```python
from build123d import *

# Parameters (mm, degrees)
BOSS_EXTRUDE1_DEPTH = 18
SKETCH2_R           = 1.75
CUT_EXTRUDE1_DEPTH  = 30.5
CUT_EXTRUDE2_DEPTH  = 1
CUT_EXTRUDE3_DEPTH  = 5


with BuildPart() as part:
    # Sketch1 → Boss-Extrude1 (new body)
    with BuildSketch(Plane(origin=(0, 0, 0), x_dir=(1, 0, 0), z_dir=(0, 1, 0))):
        with BuildLine():
            ThreePointArc((-16.998275301, 22.028571429), (-24.773162376, 20.985576383), (-31.998275301, 17.93034302))
            ThreePointArc((-31.998275301, 17.93034302), (-46.498275301, -7.471428571), (-31.998275301, -32.873200163))
            ThreePointArc((-31.998275301, -32.873200163), (-24.773162376, -35.928433526), (-16.998275301, -36.971428571))
            Line((-16.998275301, -36.971428571), (-16.998275301, -29.971428571))
            ThreePointArc((-16.998275301, -29.971428571), (-39.498275301, -7.471428571), (-16.998275301, 15.028571429))
            Line((-16.998275301, 15.028571429), (-16.998275301, 22.028571429))
        make_face()
        with BuildLine():
            Line((-16.998275301, 32.528571429), (-31.998275301, 32.528571429))
            Line((-31.998275301, 32.528571429), (-31.998275301, 17.93034302))
            ThreePointArc((-31.998275301, 17.93034302), (-24.773162376, 20.985576383), (-16.998275301, 22.028571429))
            Line((-16.998275301, 22.028571429), (-16.998275301, 32.528571429))
        make_face()
        with BuildLine():
            Line((-31.998275301, -32.873200163), (-31.998275301, -47.471428571))
            Line((-31.998275301, -47.471428571), (-16.998275301, -47.471428571))
            Line((-16.998275301, -47.471428571), (-16.998275301, -36.971428571))
            ThreePointArc((-16.998275301, -36.971428571), (-24.773162376, -35.928433526), (-31.998275301, -32.873200163))
        make_face()
    extrude(amount=BOSS_EXTRUDE1_DEPTH)

    # Sketch2 → Cut-Extrude1 (cut, through all)
    with BuildSketch(Plane(origin=(-16.998275301, 0, 0), x_dir=(0, 0, -1), z_dir=(1, 0, 0))):
        with Locations((-42.471428571, 5.25)):
            Circle(SKETCH2_R)
        with Locations((27.528571429, 5.25)):
            Circle(SKETCH2_R)
    extrude(amount=-CUT_EXTRUDE1_DEPTH, mode=Mode.SUBTRACT)

    # Sketch3 → Cut-Extrude2 (cut)
    with BuildSketch(Plane(origin=(-16.998275301, 0, 0), x_dir=(0, 0, -1), z_dir=(1, 0, 0))):
        Polygon((-40.05243206, 15.382896708), (-37.474440607, 15.382896708), (-37.474440607, 14.433110383), (-39.102645735, 14.433110383), (-39.102645735, 13.415482178), (-37.474440607, 13.415482178), (-37.474440607, 12.465695853), (-39.102645735, 12.465695853), (-39.102645735, 10.091230041), (-40.05243206, 10.091230041), align=None)
        Polygon((-35.957538563, 15.382896708), (-34.489397872, 15.382896708), (-34.489397872, 10.091230041), (-35.439184196, 10.091230041), (-35.439184196, 14.500952263), (-36.524654282, 14.500952263), align=None)
    extrude(amount=-CUT_EXTRUDE2_DEPTH, mode=Mode.SUBTRACT)

    # Sketch4 → Cut-Extrude3 (cut)
    with BuildSketch(Plane.ZY.offset(31.998275301)):
        Polygon((-26.308738524, 2.318218798), (-24.379657977, 4.840515682), (-25.599490881, 7.772296885), (-28.748404333, 8.181781202), (-30.67748488, 5.659484318), (-29.457651976, 2.727703115), align=None)
        Polygon((43.823590255, 2.376849792), (45.635730482, 4.984431264), (44.283568799, 7.857581471), (41.119266888, 8.123150208), (39.307126661, 5.515568736), (40.659288344, 2.642418529), align=None)
    extrude(amount=-CUT_EXTRUDE3_DEPTH, mode=Mode.SUBTRACT)


solid = part.part
```
The listing builds one solid part. Answer for the finished solid, in the listing's coordinates (mm). A direction names the side the tool comes from. Give positions to 0.01 mm unless a question says otherwise; leave off trailing zeros. Write each loop counter-clockwise with the first axis right and the second up, starting at its lowest first coordinate (ties: lowest second). Pieces come first, ordered by that corner, then holes. Notation, with made-up numbers: (59.25, 22.5) - (69.25, 22.5) arc R21 cw to (69.25, 40.5) - close; hole circle Ø7 at (16, 13). An arc over 180 degrees is marked (long way). Use one line per item in the form item = value. Start each with the question number.
1) The mould has two halves that part along Z. Classify faces 3 (the face through (-31.998, 9, -25)), 4 (the face through (-39.493, 8.874, 7.966)), 5 (the face through (-29.533, 4.214, -30.076)), 6 (the face through (-46.495, 8.874, 7.043)): pulls with the +Z half, pulls with the -Z half, needs draft (parallel to the pull), parting line crosses it, or undercut.
2) Flat-ended cylindrical pins translate along their axes: pin 1 Ø5 at (y, z) = (12, 1) entering from -X; pin 2 Ø4.5 at (y, z) = (9.5, -21.5) entering from -X; pin 3 Ø1.8 at (y, z) = (6.5, -27.5) entering from -X. Find the tip coordinate at first contact, or state that the pin passes through.
3) A tool of negligible diameter and unlimited length cuts with its end or side. For faces 1 (the face through (-29.53, 6.94, -29.7)), 2 (the face through (-42, 0, 7)), from which of +Z, -Z, +X, -X, +Y, -Y can it reach the whole face along a straight path? Write none if from no direction.
4) Find section C-C on y = 11.5. Determine the outline of the cut face in (x, z), plus the area to 3 significant figures.
5) Find section D-D on x = -34.5. Determine the outline of the cut face in (y, z), plus the area to 3 significant figures.
6) Find section B-B on x = -37.75. Determine the outline of the cut face in (y, z).
7) Consider line 1 along Z through (x, y) = (-25.75, 5.75); line 2 along Z through (x, y) = (-31.25, 5.5); line 3 along X through (y, z) = (15, 34). Determine where each line is inside the solid, lowest interval first. Write a range as from..to.
8) Find section A-A on x = -29.5. Determine the outline of the cut face in (y, z).
Geometry results:
q1.face_3 = needs draft
q1.face_4 = undercut
q1.face_5 = undercut
q1.face_6 = parting line crosses it
q2.pin_1 = -46.23
q2.pin_2 = -32
q2.pin_3 = -27
q3.face_1 = -X
q3.face_2 = +Z, -Z, +X, -X, -Y
q4.outline = (-32, -32.53) - (-17, -32.53) - (-17, -15.03) arc R22.5 cw to (-17, 29.97) - (-17, 34.49) - (-18, 34.49) - (-18, 35.44) - (-17, 35.44) - (-17, 39.1) - (-18, 39.1) - (-18, 40.05) - (-17, 40.05) - (-17, 47.47) - (-32, 47.47) - (-32, 32.87) arc R29.5 ccw to (-32, -17.93) - close
q4.area = 925 mm2
q5.outline = (0, -16.28) - (18, -16.28) - (18, -6.67) - (0, -6.67) - close; (0, 21.61) - (18, 21.61) - (18, 31.22) - (0, 31.22) - close
q5.area = 346 mm2
q6.outline = (0, -13.5) - (18, -13.5) - (18, -1.22) - (0, -1.22) - close; (0, 16.17) - (18, 16.17) - (18, 28.44) - (0, 28.44) - close
q7.line_1 = -32.53..-29.21, -25.85..-13.26, 28.2..40.79, 44.15..47.47
q7.line_2 = -32.53..-30.61, -24.65..-9.94, 24.88..39.31, 45.39..47.47
q7.line_3 = -32..-17
q8.outline = (0, -32.53) - (18, -32.53) - (18, -11.24) - (0, -11.24) - close; (0, 26.18) - (18, 26.18) - (18, 47.47) - (0, 47.47) - close; hole (2.32, -26.31) - (2.73, -29.46) - (5.66, -30.68) - (8.18, -28.75) - (7.77, -25.6) - (4.84, -24.38) - close; hole (2.38, 43.82) - (2.64, 40.66) - (5.52, 39.31) - (8.12, 41.12) - (7.86, 44.28) - (4.98, 45.64) - close
